Verification items for the finished model (mm, model axes). A direction names the side the tool comes from. Round coordinates to 2 decimals unless told otherwise and drop trailing zeros. Write each loop counter-clockwise with the first axis right and the second up, starting at its lowest first coordinate (ties: lowest second). Pieces come first, ordered by that corner, then holes. Notation, with made-up numbers: M 53,-5.75 L 76,-5.75 A15 cw 76,1.25 Z; hole C 35.5,72 d7. An arc over 180 degrees is marked long. Answer in a Markdown table with one row per item. Add a question column.
1. Material ranges on probe 1 along X at (y, z) = (23.5, -16); probe 2 along X at (y, z) = (29, -16); probe 3 along Z at (x, y) = (526.5, 19), recorded low to high.
2. Sectioned sample at C-C on z = -67. Record the cut outline in (x, y), plus the area to 3 significant figures.
3. Draft check along X on faces 3 (the flat face through (19, 19, -44)), 4 (the flat face through (601, 19, -88.9)), 5 (the flat face through (516, 19, -50.8)). Enter one of: pulls with the +X half, pulls with the -X half, needs draft (parallel to the pull), parting line crosses it, or undercut.
4. Go/stop test with flat-tipped pins: pin 1 Ø11.5 at (y, z) = (25, -26.5) entering from -X; pin 2 Ø1 at (y, z) = (30, -43) entering from +X; pin 3 Ø1.5 at (y, z) = (21.5, -72.5) entering from +X. Record where each tip stops, or that it passes through.
5. Sectioned sample at A-A on z = -16.5. Record the cut outline in (x, y).
6. Set-up check for faces 1 (the flat face through (884, 19, 0)), 2 (the flat face through (558.8, 19, -26)): record each of +Z, -Z, +X, -X, +Y, -Y from which the full face is reachable in a straight line by a thin tool's end or side.
7. Sectioned sample at B-B on y = 29. Record the cut outline in (x, z), plus the area to 3 significant figures.
```python
from build123d import *

# Parameters (mm, degrees)
SKETCH1_W           = 1219.2
SKETCH1_H           = 88.9
BOSS_EXTRUDE1_DEPTH = 38.1
CUT_EXTRUDE1_DEPTH  = 89.9
SKETCH3_W           = 84.1375
SKETCH3_H           = 50.8
CUT_EXTRUDE2_DEPTH  = 39.1


with BuildPart() as part:
    # Sketch1 → Boss-Extrude1 (new body)
    with BuildSketch(Plane(origin=(0, 0, 0), x_dir=(1, 0, 0), z_dir=(0, 1, 0))):
        with Locations((609.6, 44.45)):
            Rectangle(SKETCH1_W, SKETCH1_H)
    extrude(amount=BOSS_EXTRUDE1_DEPTH)

    # Sketch2 → Cut-Extrude1 (cut, through all)
    with BuildSketch(Plane.XY):
        Polygon((0, 0), (38.1, 38.1), (0, 38.1), align=None)
        Polygon((1219.2, 0), (1219.2, 38.1), (1181.1, 38.1), align=None)
    extrude(amount=-CUT_EXTRUDE1_DEPTH, mode=Mode.SUBTRACT)

    # Sketch3 → Cut-Extrude2 (cut, through all)
    with BuildSketch(Plane.XZ):
        with Locations((516.73125, -25.4)):
            Rectangle(SKETCH3_W, SKETCH3_H)
    extrude(amount=-CUT_EXTRUDE2_DEPTH, mode=Mode.SUBTRACT)


solid = part.part
```
Geometry check:
| question | item | result |
|---|---|---|
| 1 | probe 1 | x = 23.5 to 474.66, 558.8 to 1195.7 |
| 1 | probe 2 | x = 29 to 474.66, 558.8 to 1190.2 |
| 1 | probe 3 | z = -88.9 to -50.8 |
| 2 | outline | M 0,0 L 1219.2,0 L 1181.1,38.1 L 38.1,38.1 Z |
| 2 | area | 45,000 mm2 |
| 3 | face 3 | pulls with the -X half |
| 3 | face 4 | needs draft |
| 3 | face 5 | undercut |
| 4 | pin 1 | stops at x = 19.25 |
| 4 | pin 2 | stops at x = 1189.7 |
| 4 | pin 3 | stops at x = 1198.45 |
| 5 | outline | M 0,0 L 474.66,0 L 474.66,38.1 L 38.1,38.1 Z; M 558.8,0 L 1219.2,0 L 1181.1,38.1 L 558.8,38.1 Z |
| 6 | face 1 | +Z, +X, -X, +Y, -Y |
| 6 | face 2 | +Z, +Y, -Y |
| 7 | outline | M 29,-88.9 L 1190.2,-88.9 L 1190.2,0 L 558.8,0 L 558.8,-50.8 L 474.66,-50.8 L 474.66,0 L 29,0 Z |
| 7 | area | 99,000 mm2 |
